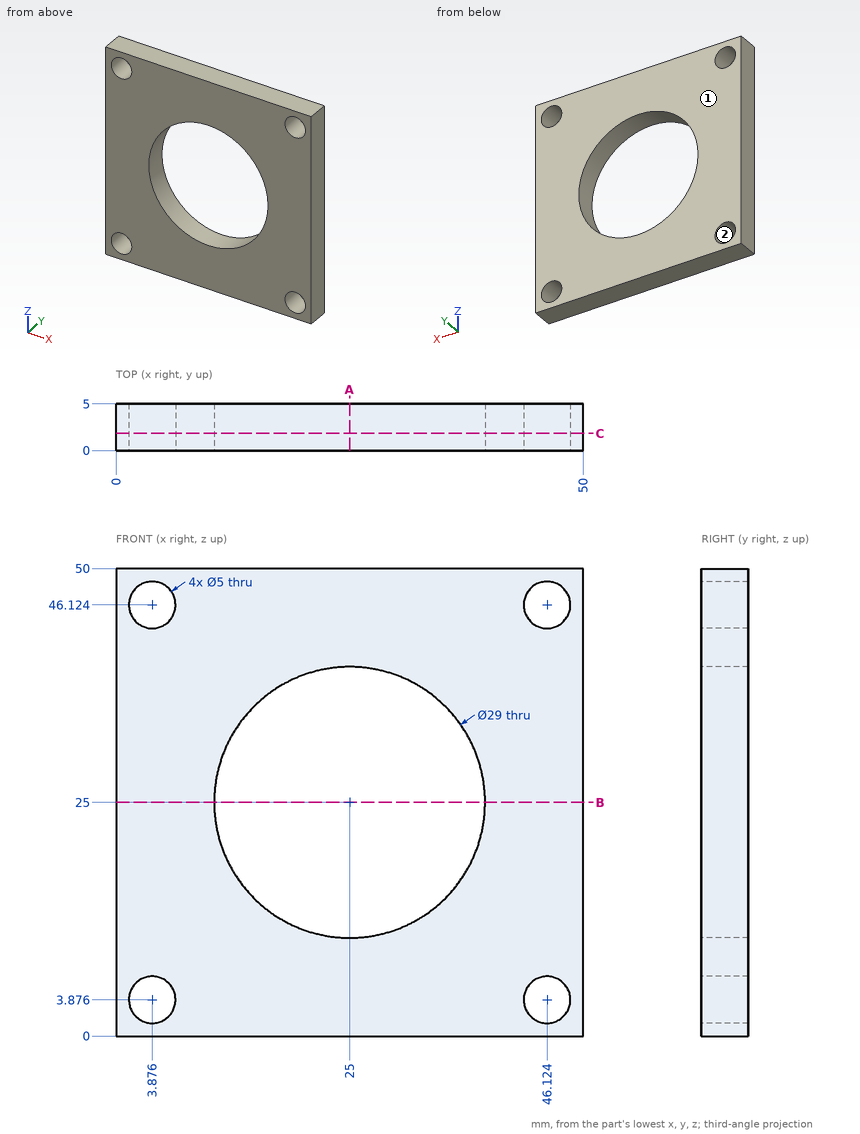
Design review of the part shown in the three views and the two pictorial views. Dimensions are in mm from the part's minimum x, y and z. Coordinates: 2 decimals unless noted, no trailing zeros. Loops run counter-clockwise (first coordinate to the right, second up) from the corner with the lowest first, then second, coordinate; pieces in that order, holes last.
(1) Consider section A-A, the plane x = 25. Give the boundary of the cut face in (y, z), plus the area to 3 significant figures.
Determined:
outline: (0, 0) - (5, 0) - (5, 10.5) - (0, 10.5) - close; (0, 39.5) - (5, 39.5) - (5, 50) - (0, 50) - close
area: 105 mm2
(2) Draft analysis for pull direction X (two halves, no side actions). For the marked faces 1 and 2, state which applies: +X half, -X half, draft (parallel to the pull), parting line (faces both ways), or undercut.
Determined:
face 1: draft
face 2: undercut
(3) Wall thickness on L1, parallel to Z at x = 25, y = 1.9; L2, parallel to X at y = 3.5, z = 46.5; L3, parallel to X at y = 0.4, z = 4.5: over which ranges is each line inside the solid? List them lowest first.
Determined:
L1: z = 0 to 10.5, 39.5 to 50
L2: x = 0 to 1.4, 6.35 to 43.65, 48.6 to 50
L3: x = 0 to 1.46, 6.3 to 43.7, 48.54 to 50
(4) Consider section C-C, the plane y = 1.85. Give the boundary of the cut face in (x, z), plus the area to 3 significant figures.
Determined:
outline: (0, 0) - (50, 0) - (50, 50) - (0, 50) - close; hole circle Ø5 at (3.88, 3.88); hole circle Ø5 at (3.88, 46.12); hole circle Ø29 at (25, 25); hole circle Ø5 at (46.12, 3.88); hole circle Ø5 at (46.12, 46.12)
area: 1,760 mm2
(5) Consider section B-B, the plane z = 25. Give the boundary of the cut face in (x, y).
Determined:
outline: (0, 0) - (10.5, 0) - (10.5, 5) - (0, 5) - close; (39.5, 0) - (50, 0) - (50, 5) - (39.5, 5) - close
(6) Insertion check: P1, Ø3, axis at x = 46.124, z = 3.876, coming from the +Y side. The pin has a flat end and moves straight along its axis. Give the tip position at first contact, or say it passes through.
Determined:
P1: passes through
